Build history of the part. All positions in model axes, mm. Give positions to 0.01 mm unless a question says otherwise; leave off trailing zeros. Order: outer loops, then holes, each group sorted by start corner. A loop starts at its lowest first (then second) coordinate and runs counter-clockwise, first axis right, second up. Notation, with made-up numbers: M -12.5,-23 L -5.5,-23 A33 cw -5.5,6 Z; hole C 39.25,44 d3. An arc over 180 degrees is marked long. One line per item, written item: value. Start each with the question number.
Autodesk Inventor part; units mm, degrees
ref_plane "YZ Plane" through (0, 0, 0) normal (1, 0, 0) x (0, 1, 0)
ref_plane "XZ Plane" through (0, 0, 0) normal (0, 1, 0) x (-1, 0, 0)
ref_plane "XY Plane" through (0, 0, 0) normal (0, 0, 1) x (1, 0, 0)
sketch "スケッチ1" plane through (0, 0, 0) normal (0, 0, 1) x (1, 0, 0)
  circle A0 centre (0, 0) radius 5.985
  circle A1 centre (0, 8.5) radius 1.35
  line L0 (0, 8.5) -> (0, 0) construction
  circle A2 centre (0, 0) radius 8.5 construction
  circle A3 centre (0, 0) radius 10.5 construction
  arc A4 (2.5, 8.124) -> (-2.5, 8.124) centre (0, 7.9968) ccw
  arc A5 (-8.124, 2.5) -> (-8.124, -2.5) centre (-7.9968, 0) ccw
  circle A6 centre (-8.5, 0) radius 1.35
  arc A7 (-2.5, -8.124) -> (2.5, -8.124) centre (0, -7.9968) ccw
  circle A8 centre (0, -8.5) radius 1.35
  arc A9 (8.124, -2.5) -> (8.124, 2.5) centre (7.9968, 0) ccw
  circle A10 centre (8.5, 0) radius 1.35
  arc A11 (-2.5, 8.124) -> (-8.124, 2.5) centre (0, 0) ccw
  arc A12 (-8.124, -2.5) -> (-2.5, -8.124) centre (0, 0) ccw
  arc A13 (2.5, -8.124) -> (8.124, -2.5) centre (0, 0) ccw
  arc A14 (8.124, 2.5) -> (2.5, 8.124) centre (0, 0) ccw
  point P0 (0, 10.5)
  point P1 (-10.5, 0)
  point P2 (0, -10.5)
  point P3 (10.5, 0)
  dimension "d39" = 21
  dimension "d1" = 11.97
  dimension "d2" = 2.7
  dimension "d5" = 17
  dimension "d40" = 5
  dimension "d43" = 360
extrude "押し出し1" add sketch "スケッチ1" along normal blind 5
fillet "フィレット1" radius 2 8 edges at (-8.124, -2.5, 2.5) (-2.5, -8.124, 2.5) (2.5, -8.124, 2.5) (8.124, -2.5, 2.5) (8.124, 2.5, 2.5) (2.5, 8.124, 2.5) (-2.5, 8.124, 2.5) (-8.124, 2.5, 2.5)
properties part number "Knee_clamp" material "アルミニウム 2014-T4"
1) Drill centre lines: line 1 (Y direction, x = 0, z = 3.3) (3 decimals); line 2 (X direction, y = -1, z = 2.25); line 3 (X direction, y = 0.5, z = 4.35). Where is each one in solid material? Low to high.
2) Slice it at C-C (x = 5.5). List the corners of the cut face in (y, z), plus the area to 3 significant figures.
3) Slice it at A-A (x = 0). List the corners of the cut face in (y, z) (3 decimals).
4) Drop flat-ended pins along their axis: P1, Ø1.5, axis at y = 7.5, z = 2, coming from the +X side; P2, Ø2, axis at x = 4.5, z = 2, coming from the +Y side; P3, Ø2, axis at x = -2, z = 3.5, coming from the +Y side. Give the stop position or say it passes through.
5) Pull direction Y, two halves, no side cores. Call faces 1 (the cylindrical face through (-0.176, 7.161, 2.465)), 2 (the cylindrical face through (-6.04, 5.98, 2.46)), 3 (the flat face through (-5, 4, 5)), 4 (the cylindrical face through (-1.297, 5.843, 2.465)): pulls with the +Y half, pulls with the -Y half, needs draft (parallel to the pull), parting line crosses it, or undercut.
6) Slice it at D-D (z = 0.85). State how many separate pieces and enclosed holes the cut face has, plus the area to 3 significant figures.
Results list:
1. line 1: y = -10.5 to -9.85, -7.15 to -5.985, 5.985 to 7.15, 9.85 to 10.5
1. line 2: x = -10.29 to -9.41, -7.59 to -5.9, 5.9 to 7.59, 9.41 to 10.29
1. line 3: x = -10.45 to -9.75, -7.25 to -5.96, 5.96 to 7.25, 9.75 to 10.45
2. outline: M -6.48,0 L -2.36,0 L -2.36,5 L -6.48,5 Z; M 2.36,0 L 6.48,0 L 6.48,5 L 2.36,5 Z
2. area: 41.2 mm²
3. outline: M -10.5,0 L -9.85,0 L -9.85,5 L -10.5,5 Z; M -7.15,0 L -5.985,0 L -5.985,5 L -7.15,5 Z; M 5.985,0 L 7.15,0 L 7.15,5 L 5.985,5 Z; M 9.85,0 L 10.5,0 L 10.5,5 L 9.85,5 Z
4. P1: stops at x = 5.17
4. P2: stops at y = 7.75
4. P3: stops at y = 10.29
5. face 1: undercut
5. face 2: pulls with the +Y half
5. face 3: needs draft
5. face 4: undercut
6. separate pieces: 1
6. enclosed holes: 5
6. area: 124 mm²
